from build123d import *

# Parameters (mm, degrees)
SKETCH_1_R      = 1.05
EXTRUDE_1_DEPTH = 5.5
FILLET_1_R      = 3
FILLET_2_R      = 2


with BuildPart() as part:
    # ｽｹｯﾁ1 → ﾎﾞｽ - 押し出し1 (new body)
    with BuildSketch(Plane.XY):
        Polygon((0, 0), (13, 0), (7, 10), (0, 10), align=None)
        with Locations((3, 3)):
            Circle(SKETCH_1_R, mode=Mode.SUBTRACT)
        with Locations((8, 3)):
            Circle(SKETCH_1_R, mode=Mode.SUBTRACT)
    extrude(amount=EXTRUDE_1_DEPTH)

    # ﾌｨﾚｯﾄ1
    fillet_1_edges = [part.edges().sort_by_distance(p)[0] for p in [
        (13, 0, 2.75),
    ]]
    fillet(fillet_1_edges, radius=FILLET_1_R)

    # ﾌｨﾚｯﾄ2
    fillet_2_edges = [part.edges().sort_by_distance(p)[0] for p in [
        (0, 10, 2.75),
        (7, 10, 2.75),
        (0, 0, 2.75),
    ]]
    fillet(fillet_2_edges, radius=FILLET_2_R)


solid = part.part
Check sheet for the modelled part. Datum: model origin and axes. Units: mm. Round coordinates to 2 decimals unless told otherwise and drop trailing zeros. Order: outer loops, then holes, each group sorted by start corner. A loop starts at its lowest first (then second) coordinate and runs counter-clockwise, first axis right, second up.
(1) Cross-section at D-D, the plane y = 5.25. Enter the section's corners in (x, z).
(2) Scan lines: probe 1 along X at (y, z) = (2.75, 3.75); probe 2 along Y at (x, z) = (3, 4); probe 3 along X at (y, z) = (5, 0.55). Record each from-to range of solid material in increasing order.
(3) Cross-section at B-B, the plane z = 0.55. Enter the section's corners in (x, y).
(4) Cross-section at A-A, the plane y = 3. Enter the section's corners in (x, z).
(5) Cross-section at C-C, the plane x = 3.25. Enter the section's corners in (y, z), and give its area (3 significant figures).
(6) Draft check along X on faces 1 (the cylindrical face through (6.87, 9.73, 2.79)), 2 (the cylindrical face through (7.86, 4.04, 2.71)), 3 (the flat face through (4, 10, 3)). Enter one of: pulls with the +X half, pulls with the -X half, needs draft (parallel to the pull), parting line crosses it, or undercut.
(7) Go/stop test with a flat-tipped pin: P1, Ø2, axis at y = 6.5, z = 3.5, coming from the +X side. Record where the tip stops, or that it passes through.
Check sheet entries:
1. outline: (0, 0) - (9.85, 0) - (9.85, 5.5) - (0, 5.5) - close
2. probe 1: x = 0 to 1.98, 4.02 to 6.98, 9.02 to 10.69
2. probe 2: y = 0 to 1.95, 4.05 to 10
2. probe 3: x = 0 to 10
3. outline: (0, 2) arc R2 ccw to (2, 0) - (7.7, 0) arc R3 ccw to (10.27, 4.54) - (7.58, 9.03) arc R2 ccw to (5.87, 10) - (2, 10) arc R2 ccw to (0, 8) - close; hole circle Ø2.1 at (3, 3); hole circle Ø2.1 at (8, 3)
4. outline: (0, 0) - (1.95, 0) - (1.95, 5.5) - (0, 5.5) - close; (4.05, 0) - (6.95, 0) - (6.95, 5.5) - (4.05, 5.5) - close; (9.05, 0) - (10.7, 0) - (10.7, 5.5) - (9.05, 5.5) - close
5. outline: (0, 0) - (1.98, 0) - (1.98, 5.5) - (0, 5.5) - close; (4.02, 0) - (10, 0) - (10, 5.5) - (4.02, 5.5) - close
5. area: 43.8 mm2
6. face 1: pulls with the +X half
6. face 2: undercut
6. face 3: needs draft
7. P1: stops at x = 9.7
